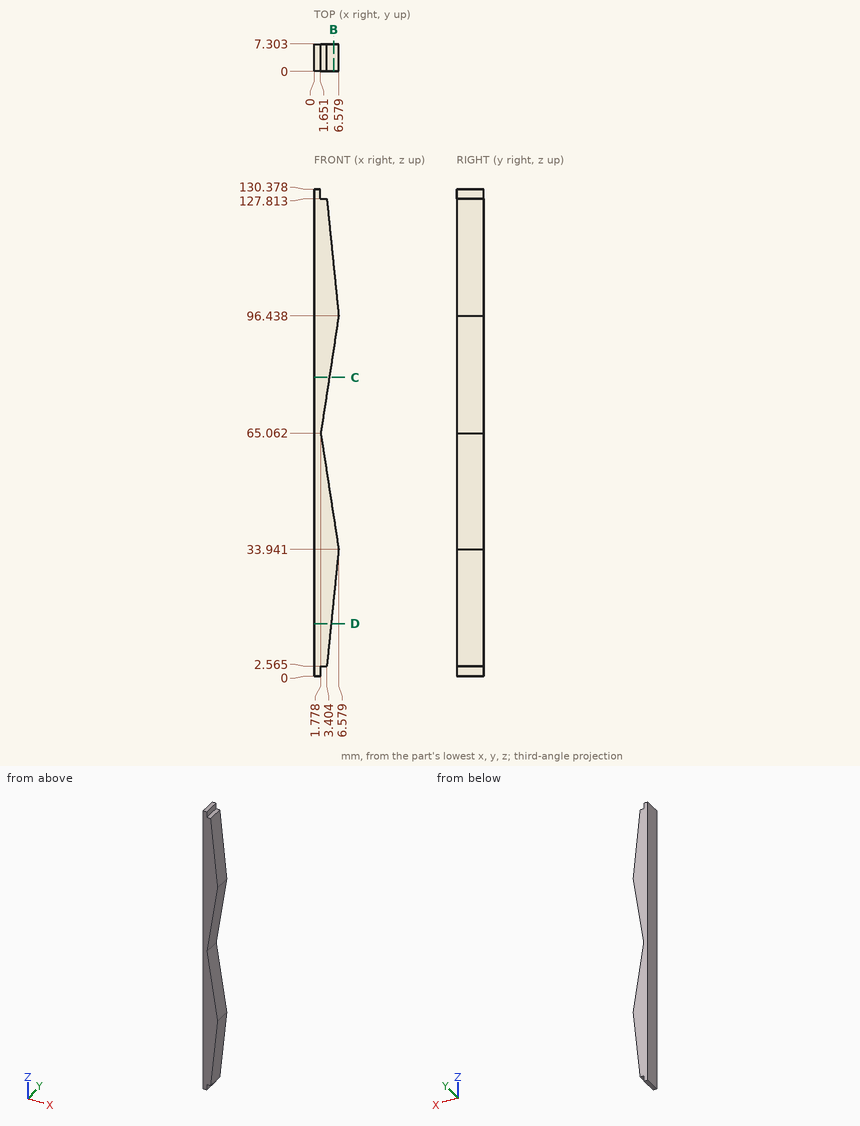
Print and shaded views of the part. All mm, measured from the part's lowest x, y and z. Coordinates: 2 decimals unless noted, no trailing zeros. Loops run counter-clockwise (first coordinate to the right, second up) from the corner with the lowest first, then second, coordinate; pieces in that order, holes last. Notation, with made-up numbers: (-28, 26) -> (-16, 26) arc R22 ccw to (-16, 40) -> close; hole circle Ø7 at (53, 17). An arc over 180 degrees is marked (long way). Use one line per item in the form item = value. Start each with the question number.
(1) Cut at D-D on z = 14. Give the cut face in (x, y).
(2) Flat gauge pins, fed straight in: pin 1 (0.5 mm diameter, centred on x = 3, y = 3.5, fed in from +Z); pin 2 (1.3 mm diameter, centred on y = 4.5, z = 129.5, fed in from +X); pin 3 (0.5 mm diameter, centred on x = 3, y = 3, fed in from -Z) (1 decimal). Where does each tip first touch, or does it go through?
(3) Cut at C-C on z = 80. Give the cut face in (x, y).
(4) Cut at B-B on x = 5.25. Give the cut face in (y, z) (1 decimal), and give its area (3 significant figures).
(5) Probe probe 1 along X at (y, z) = (2.5, 105); probe 2 along X at (y, z) = (5.5, 15.5). List the from-to ranges inside material, lowest first. Write a range as from..to.
Values:
q1.outline = (0, 0) -> (4.56, 0) -> (4.56, 7.3) -> (0, 7.3) -> close
q2.pin_1 = 127.81
q2.pin_2 = 1.65
q2.pin_3 = 2.6
q3.outline = (0, 0) -> (4.06, 0) -> (4.06, 7.3) -> (0, 7.3) -> close
q4.outline = (0, 20.8) -> (7.3, 20.8) -> (7.3, 42.6) -> (0, 42.6) -> close; (0, 87.8) -> (7.3, 87.8) -> (7.3, 109.6) -> (0, 109.6) -> close
q4.area = 318 mm2
q5.probe_1 = 0..5.71
q5.probe_2 = 0..4.71
